Geometry: final body of the model. Coordinates: model frame, mm. A direction names the side the tool comes from. Coordinates: 2 decimals unless noted, no trailing zeros. Write each loop counter-clockwise with the first axis right and the second up, starting at its lowest first coordinate (ties: lowest second). Pieces come first, ordered by that corner, then holes. Notation, with made-up numbers: (30.25, 88.25) -> (56.25, 88.25) arc R22 ccw to (56.25, 104.25) -> close; hole circle Ø1 at (-38, 57). An arc over 180 degrees is marked (long way). One line per item, written item: value.
Autodesk Inventor part; units mm, degrees
ref_plane "YZ Plane" through (0, 0, 0) normal (1, 0, 0) x (0, 1, 0)
ref_plane "XZ Plane" through (0, 0, 0) normal (0, 1, 0) x (-1, 0, 0)
ref_plane "XY Plane" through (0, 0, 0) normal (0, 0, 1) x (1, 0, 0)
sketch "Sketch1" plane through (0, 0, 0) normal (0, 0, 1) x (1, 0, 0)
  line L0 (3.935, -2.2719) -> (0, -4.5437)
  line L1 (0, -4.5437) -> (-3.935, -2.2719)
  line L2 (-3.935, -2.2719) -> (-3.935, 2.2719)
  line L3 (-3.935, 2.2719) -> (0, 4.5437)
  line L4 (0, 4.5437) -> (3.935, 2.2719)
  line L5 (3.935, 2.2719) -> (3.935, -2.2719)
  circle A0 centre (0.79, 0) radius 2.5
  point P0 (0, 0)
  point P1 (0, 0)
  dimension "d0" = 7.87
  dimension "d1" = 0.79
  dimension "d2" = 5
extrude "Extrusion1" add sketch "Sketch1" along normal blind 6.35
sketch "Sketch2" plane through (0, 0, 6.35) normal (0, 0, 1) x (1, 0, 0)
  circle A0 centre (0.79, 0) radius 2.5
  circle A1 centre (0, 0) radius 3.555
  dimension "d5" = 7.11
extrude "Extrusion2" add sketch "Sketch2" along normal blind 1.27
sketch "Sketch3" plane through (3.935, -2.2719, 0) normal (1, 0, 0) x (0, 0, -1)
  circle A0 centre (-3.175, 2.2719) radius 1
  point P0 (0, 2.2719)
  dimension "d8" = 2
extrude "Extrusion3" cut sketch "Sketch3" against normal blind 0.15
properties part number "Eccentric M5 Spacer" material "Stainless Steel"
(1) Reachability of faces 5 (the cylindrical face through (3.39, -1.07, 6.98)), 6 (the flat face through (1.94, 3.424, 3.131)) from +Z, -Z, +X, -X, +Y, -Y: full face, straight path, thin tool, end or side. Return the list, or none.
Responses:
face 5: +Z
face 6: +Z, -Z, +X, +Y
(2) Line query: line 1 (Z direction, x = -2.75, y = -2.75); line 2 (X direction, y = -1, z = 5.75) (3 decimals); line 3 (X direction, y = 0.5, z = 6.25) (3 decimals). Output: solid intervals per line, ascending. Write a range as [from, to].
Responses:
line 1: z = [0, 6.35]
line 2: x = [-3.935, -1.501], [3.081, 3.935]
line 3: x = [-3.935, -1.659], [3.239, 3.935]
(3) Section B-B (z = 4.5). Return the cut outline in (x, y) (3 decimals).
Responses:
outline: (-3.935, -2.272) -> (0, -4.544) -> (3.935, -2.272) -> (3.935, 2.272) -> (0, 4.544) -> (-3.935, 2.272) -> close; hole circle Ø5 at (0.79, 0)
(4) First-contact query: pin 1 (4.5 mm diameter, centred on x = 0.79, y = 0, fed in from +Z); pin 2 (1 mm diameter, centred on x = 1.5, z = 5, fed in from +Y). Flat tips, straight axial feed; report the tip coordinate or a pass-through.
Responses:
pin 1: passes through
pin 2: stops at y = 3.97
(5) Section C-C (x = -1.25). Return the cut outline in (y, z).
Responses:
outline: (-3.82, 0) -> (-1.45, 0) -> (-1.45, 7.62) -> (-3.33, 7.62) -> (-3.33, 6.35) -> (-3.82, 6.35) -> close; (1.45, 0) -> (3.82, 0) -> (3.82, 6.35) -> (3.33, 6.35) -> (3.33, 7.62) -> (1.45, 7.62) -> close
(6) Section D-D (z = 2.75). Return the cut outline in (x, y) (3 decimals), then the cut area to 3 significant figures.
Responses:
outline: (-3.935, -2.272) -> (0, -4.544) -> (3.935, -2.272) -> (3.935, -0.905) -> (3.785, -0.905) -> (3.785, 0.905) -> (3.935, 0.905) -> (3.935, 2.272) -> (0, 4.544) -> (-3.935, 2.272) -> close; hole circle Ø5 at (0.79, 0)
area: 33.7 mm2
(7) Section A-A (y = 0). Return the cut outline in (x, z) (3 decimals).
Responses:
outline: (-3.935, 0) -> (-1.71, 0) -> (-1.71, 7.62) -> (-3.555, 7.62) -> (-3.555, 6.35) -> (-3.935, 6.35) -> close; (3.29, 0) -> (3.935, 0) -> (3.935, 2.175) -> (3.785, 2.175) -> (3.785, 4.175) -> (3.935, 4.175) -> (3.935, 6.35) -> (3.555, 6.35) -> (3.555, 7.62) -> (3.29, 7.62) -> close
(8) Pull-direction query (Z, two-part tool) for faces 1 (the flat face through (-1.94, -3.424, 3.131)), 2 (the flat face through (-2, 0, 0)), 3 (the flat face through (3.785, 0, 3)), 4 (the flat face through (0, -4, 6.35)); classes: released by +Z, released by -Z, zero draft, split by the parting line, or undercut.
Responses:
face 1: zero draft
face 2: released by -Z
face 3: undercut
face 4: released by +Z
